```python
from build123d import *

# Parameters (mm, degrees)
SKETCH1_W             = 3
SKETCH1_H             = 3
BOSS_EXTRUDE1_DEPTH   = 8
BOSS_EXTRUDE1_2_DEPTH = 8
BOSS_EXTRUDE1_3_DEPTH = 8
BOSS_EXTRUDE1_4_DEPTH = 8
SKETCH2_W             = 30
SKETCH2_H             = 15
BOSS_EXTRUDE2_DEPTH   = 3
CUT_EXTRUDE1_DEPTH    = 21.05617112
CUT_EXTRUDE2_DEPTH    = 21.05617112
BOSS_EXTRUDE3_DEPTH   = 2
CHAMFER1_SIZE         = 1.25
SKETCH7_W             = 3
SKETCH7_H             = 3
BOSS_EXTRUDE4_DEPTH   = 3


with BuildPart() as part:
    # Sketch1 → Boss-Extrude1 (new body)
    with BuildSketch(Plane(origin=(0, 0, 0), x_dir=(1, 0, 0), z_dir=(0, 1, 0))):
        with Locations((-13.5, 6)):
            Rectangle(SKETCH1_W, SKETCH1_H)
    extrude(amount=BOSS_EXTRUDE1_DEPTH)



with BuildPart() as body_2:
    # Sketch1 → Boss-Extrude1 2 (new body)
    with BuildSketch(Plane(origin=(0, 0, 0), x_dir=(1, 0, 0), z_dir=(0, 1, 0))):
        with Locations((13.5, 6)):
            Rectangle(SKETCH1_W, SKETCH1_H)
    extrude(amount=BOSS_EXTRUDE1_2_DEPTH)


with BuildPart() as body_3:
    # Sketch1 → Boss-Extrude1 3 (new body)
    with BuildSketch(Plane(origin=(0, 0, 0), x_dir=(1, 0, 0), z_dir=(0, 1, 0))):
        with Locations((13.5, -6)):
            Rectangle(SKETCH1_W, SKETCH1_H)
    extrude(amount=BOSS_EXTRUDE1_3_DEPTH)


with BuildPart() as body_4:
    # Sketch1 → Boss-Extrude1 4 (new body)
    with BuildSketch(Plane(origin=(0, 0, 0), x_dir=(1, 0, 0), z_dir=(0, 1, 0))):
        with Locations((-13.5, -6)):
            Rectangle(SKETCH1_W, SKETCH1_H)
    extrude(amount=BOSS_EXTRUDE1_4_DEPTH)


with BuildPart() as part_1:
    add(part.part)

    add(body_2.part)  # Boss-Extrude2 merges body 2

    add(body_3.part)  # Boss-Extrude2 merges body 3

    add(body_4.part)  # Boss-Extrude2 merges body 4
    # Sketch2 → Boss-Extrude2 (add)
    with BuildSketch(Plane(origin=(0, 8, 0), x_dir=(1, 0, 0), z_dir=(0, 1, 0))):
        Rectangle(SKETCH2_W, SKETCH2_H)
    extrude(amount=BOSS_EXTRUDE2_DEPTH)

    # Sketch3 → Cut-Extrude1 (cut, through all)
    with BuildSketch(Plane(origin=(0, 11, 0), x_dir=(1, 0, 0), z_dir=(0, 1, 0))):
        Polygon((-12, 7.5), (-9, 4.5), (9, 4.5), (12, 7.5), align=None)
        Polygon((-12, -7.5), (-9, -4.5), (9, -4.5), (12, -7.5), align=None)
        Polygon((-15, 4.5), (-12, 1.5), (-12, -1.5), (-15, -4.5), align=None)
        Polygon((15, 4.5), (12, 1.5), (12, -1.5), (15, -4.5), align=None)
    extrude(amount=-CUT_EXTRUDE1_DEPTH, mode=Mode.SUBTRACT)

    # Sketch4 → Cut-Extrude2 (cut, through all)
    with BuildSketch(Plane(origin=(0, 11, 0), x_dir=(1, 0, 0), z_dir=(0, 1, 0))):
        with BuildLine():
            Line((-8, 1.75), (8, 1.75))
            ThreePointArc((8, 1.75), (8.707106781, 1.457106781), (9, 0.75))
            Line((9, 0.75), (9, -0.75))
            ThreePointArc((9, -0.75), (8.707106781, -1.457106781), (8, -1.75))
            Line((8, -1.75), (-8, -1.75))
            ThreePointArc((-8, -1.75), (-8.707106781, -1.457106781), (-9, -0.75))
            Line((-9, -0.75), (-9, 0.75))
            ThreePointArc((-9, 0.75), (-8.707106781, 1.457106781), (-8, 1.75))
        make_face()
    extrude(amount=-CUT_EXTRUDE2_DEPTH, mode=Mode.SUBTRACT)

    # Sketch6 → Boss-Extrude3 (add)
    with BuildSketch(Plane.XZ):
        Polygon((-10.75, 7.5), (-12, 7.5), (-12, 4.5), (-15, 4.5), (-15, 3.25), (-10.75, 3.25), align=None)
        Polygon((12, 4.5), (12, 7.5), (10.75, 7.5), (10.75, 3.25), (15, 3.25), (15, 4.5), align=None)
        Polygon((10.75, -7.5), (12, -7.5), (12, -4.5), (15, -4.5), (15, -3.25), (10.75, -3.25), align=None)
        Polygon((-12, -4.5), (-12, -7.5), (-10.75, -7.5), (-10.75, -3.25), (-15, -3.25), (-15, -4.5), align=None)
    extrude(amount=-BOSS_EXTRUDE3_DEPTH)

    # Chamfer1
    chamfer1_edges = [part_1.edges().sort_by_distance(p)[0] for p in [
        (-12, 2, 6),
        (-13.5, 2, 4.5),
        (-13.5, 2, -4.5),
        (-12, 2, -6),
        (12, 2, 6),
        (13.5, 2, 4.5),
        (12, 2, -6),
        (13.5, 2, -4.5),
    ]]
    chamfer(chamfer1_edges, length=CHAMFER1_SIZE - 0.0001)  # a hair under: the kernel refuses the full size

    # Sketch7 → Boss-Extrude4 (add)
    with BuildSketch(Plane.XZ):
        with Locations((-13.5, 6)):
            Rectangle(SKETCH7_W, SKETCH7_H)
        with Locations((-13.5, -6)):
            Rectangle(SKETCH7_W, SKETCH7_H)
        with Locations((13.5, -6)):
            Rectangle(SKETCH7_W, SKETCH7_H)
        with Locations((13.5, 6)):
            Rectangle(SKETCH7_W, SKETCH7_H)
    extrude(amount=BOSS_EXTRUDE4_DEPTH)


solid = part_1.part
```
CAD build for the part. Positions are in the model's coordinates, mm. A direction names the side the tool comes from. Coordinates: 2 decimals unless noted, no trailing zeros. Write each loop counter-clockwise with the first axis right and the second up, starting at its lowest first coordinate (ties: lowest second). Pieces come first, ordered by that corner, then holes.
(1) Two-plate mould, pull along Y, no slides. Class faces 1 (the face through (12, 10, 0)), 2 (the face through (13, -3, 6)), 3 (the face through (-12, 6, -6)): +Y half, -Y half, draft (parallel to the pull), parting line (faces both ways), or undercut.
(2) Drill centre lines: probe 1 along X at (y, z) = (5.5, 6.5); probe 2 along X at (y, z) = (10, 0.5); probe 3 along Y at (x, z) = (-1, -2). Where is each one in solid material? Low to high.
(3) Cut at A-A, the plane x = 3.5. List the corners of the cut face in (y, z), and give its area (3 significant figures).
(4) Cut at C-C, the plane y = 5.5. List the corners of the cut face in (x, z), and give its area (3 significant figures).
(5) Flat gauge pins, fed straight in: pin 1 (2 mm diameter, centred on x = -10.5, y = 8, fed in from +Z); pin 2 (1 mm diameter, centred on x = -2.5, z = -2, fed in from -Y); pin 3 (0.9 mm diameter, centred on y = 9, z = 0, fed in from -X); pin 4 (8 mm diameter, centred on x = -3, z = 5.5, fed in from +Y). Where does each tip first touch, or does it go through?
(6) Cut at D-D, the plane y = 9. List the corners of the cut face in (x, z).
(7) 3-axis set-ups, long thin cutter, end or side, ignore diameter. For faces 4 (the face through (-13.5, 9.5, -3)), 5 (the face through (0, 10, 1.75)), 6 (the face through (11.38, 2.63, 5.82)), 7 (the face through (-12, 10, 0)), 8 (the face through (-10.75, 1, -5)): which of +Z, -Z, +X, -X, +Y, -Y reach the whole face in a straight line?
(8) Cut at B-B, the plane z = 0. List the corners of the cut face in (x, y), and give its area (3 significant figures).
Geometry says:
1. face 1: draft
1. face 2: -Y half
1. face 3: undercut
2. probe 1: x = -15 to -12, 12 to 15
2. probe 2: x = -12 to -9, 9 to 12
2. probe 3: y = 8 to 11
3. outline: (8, -4.5) - (11, -4.5) - (11, -1.75) - (8, -1.75) - close; (8, 1.75) - (11, 1.75) - (11, 4.5) - (8, 4.5) - close
3. area: 16.5 mm2
4. outline: (-15, -7.5) - (-12, -7.5) - (-12, -4.5) - (-15, -4.5) - close; (-15, 4.5) - (-12, 4.5) - (-12, 7.5) - (-15, 7.5) - close; (12, -7.5) - (15, -7.5) - (15, -4.5) - (12, -4.5) - close; (12, 4.5) - (15, 4.5) - (15, 7.5) - (12, 7.5) - close
4. area: 36.0 mm2
5. pin 1: stops at z = 7
5. pin 2: stops at y = 8
5. pin 3: stops at x = -12
5. pin 4: stops at y = 11
6. outline: (-15, -7.5) - (-12, -7.5) - (-9, -4.5) - (9, -4.5) - (12, -7.5) - (15, -7.5) - (15, -4.5) - (12, -1.5) - (12, 1.5) - (15, 4.5) - (15, 7.5) - (12, 7.5) - (9, 4.5) - (-9, 4.5) - (-12, 7.5) - (-15, 7.5) - (-15, 4.5) - (-12, 1.5) - (-12, -1.5) - (-15, -4.5) - close; hole (-9, -0.75) arc R1 ccw to (-8, -1.75) - (8, -1.75) arc R1 ccw to (9, -0.75) - (9, 0.75) arc R1 ccw to (8, 1.75) - (-8, 1.75) arc R1 ccw to (-9, 0.75) - close
7. face 4: -X, +Y
7. face 5: +Y, -Y
7. face 6: +Z, -Z
7. face 7: -X, +Y, -Y
7. face 8: +Z, -Z, -Y
8. outline: (-12, 8) - (-9, 8) - (-9, 11) - (-12, 11) - close; (9, 8) - (12, 8) - (12, 11) - (9, 11) - close
8. area: 18.0 mm2
